```python
from build123d import *

# Parameters (mm, degrees)
F0_W     = 20.32
F0_H     = 10.16
F1_DEPTH = 5.08
F2_W     = 10.5029
F2_H     = 10.16
F3_DEPTH = 2.54
F5_D     = 1.27
F7_R     = 2.75
F7_R_2   = 0.635
F8_DEPTH = 1.524


with BuildPart() as f1:
    # F0 (on Top) → F1 (new body)
    with BuildSketch(Plane.XY):
        Rectangle(F0_W, F0_H)
    extrude(amount=F1_DEPTH)

    # F2 (on face) → F3 (cut)
    with BuildSketch(Plane.XY.offset(5.08)):
        with Locations((-2.36855, 0)):
            Rectangle(F2_W, F2_H)
    extrude(amount=-F3_DEPTH, mode=Mode.SUBTRACT)

    # F5 (through all)
    with Locations(Plane.XY.offset(5.08)):
        with Locations((6.35, 1.27), (6.35, -1.27)):
            Hole(F5_D / 2)

    # F7 (on face) → F8 (cut)
    with BuildSketch(Plane(origin=(0, 0, 0), x_dir=(1, 0, 0), z_dir=(0, 0, -1))):
        with Locations((6.35, 0)):
            Circle(F7_R)
        with Locations((6.35, -1.27)):
            Circle(F7_R_2, mode=Mode.SUBTRACT)
        with Locations((6.35, 1.27)):
            Circle(F7_R_2, mode=Mode.SUBTRACT)
    extrude(amount=-F8_DEPTH, mode=Mode.SUBTRACT)


solid = f1.part
```
CAD build for the part. Positions are in the model's coordinates, mm. A direction names the side the tool comes from. Give positions to 0.01 mm unless a question says otherwise; leave off trailing zeros. Write each loop counter-clockwise with the first axis right and the second up, starting at its lowest first coordinate (ties: lowest second). Pieces come first, ordered by that corner, then holes. Notation, with made-up numbers: M 28.25,24.25 L 61.25,24.25 A22 cw 61.25,62.25 Z; hole C 53.5,-23.5 d9. An arc over 180 degrees is marked long. Return JSON: item names as keys, results as strings. Group by question number.
(1) 3-axis set-ups, long thin cutter, end or side, ignore diameter. For faces 5 (the face through (-10.16, 0, 3)), 6 (the face through (-2, 0, 2.54)), 7 (the face through (3.6, -0.1, 0.8)): which of +Z, -Z, +X, -X, +Y, -Y reach the whole face in a straight line?
(2) Band-saw the part on A-A (z = 3). Give the cut face in (x, y) (3 decimals).
(3) Flat gauge pins, fed straight in: pin 1 Ø4.5 at (x, y) = (6, 0) entering from -Z; pin 2 Ø5 at (x, y) = (-2.5, 0) entering from +Z; pin 3 Ø1.1 at (x, y) = (6.35, 1.27) entering from -Z. Where does each tip first touch, or does it go through?
(4) Mould opens along X. For faces 1 (the face through (6, 0, 5.08)), 2 (the face through (6.984, -1.242, 3.277)), 3 (the face through (2.883, 0, 4)), 4 (the face through (10.16, 0, 3)) say: pulls with the +X half, pulls with the -X half, needs draft (parallel to the pull), parting line crosses it, or undercut.
(5) Band-saw the part on C-C (y = 4.5). Give the cut face in (x, z).
(6) Band-saw the part on D-D (y = -1.5). Give the cut face in (x, z).
(7) Band-saw the part on B-B (x = 6.35). Give the cut face in (y, z) (3 decimals).
(8) Drill centre lines: L1, parallel to X at y = 1.25, z = 4.65; L2, parallel to Y at x = 6.35, z = 2.85 (3 decimals); L3, parallel to X at y = 0, z = 0.6. Where is each one in solid material? Low to high. Write a range as [from, to].
Entries:
{
 "1": {"face 5": "+Z, -Z, -X, +Y, -Y", "face 6": "+Z, +Y, -Y", "face 7": "-Z"},
 "2": {"outline": "M -10.16,-5.08 L -7.62,-5.08 L -7.62,5.08 L -10.16,5.08 Z; M 2.883,-5.08 L 10.16,-5.08 L 10.16,5.08 L 2.883,5.08 Z; hole C 6.35,-1.27 d1.27; hole C 6.35,1.27 d1.27"},
 "3": {"pin 1": "stops at z = 1.52", "pin 2": "stops at z = 2.54", "pin 3": "passes through"},
 "4": {"face 1": "needs draft", "face 2": "undercut", "face 3": "undercut", "face 4": "pulls with the +X half"},
 "5": {"outline": "M -10.16,0 L 10.16,0 L 10.16,5.08 L 2.88,5.08 L 2.88,2.54 L -7.62,2.54 L -7.62,5.08 L -10.16,5.08 Z"},
 "6": {"outline": "M -10.16,0 L 4.05,0 L 4.05,1.52 L 5.76,1.52 L 5.76,5.08 L 2.88,5.08 L 2.88,2.54 L -7.62,2.54 L -7.62,5.08 L -10.16,5.08 Z; M 6.94,1.52 L 8.65,1.52 L 8.65,0 L 10.16,0 L 10.16,5.08 L 6.94,5.08 Z"},
 "7": {"outline": "M -5.08,0 L -2.75,0 L -2.75,1.524 L -1.905,1.524 L -1.905,5.08 L -5.08,5.08 Z; M -0.635,1.524 L 0.635,1.524 L 0.635,5.08 L -0.635,5.08 Z; M 1.905,1.524 L 2.75,1.524 L 2.75,0 L 5.08,0 L 5.08,5.08 L 1.905,5.08 Z"},
 "8": {"L1": "x = [-10.16, -7.62], [2.88, 5.72], [6.98, 10.16]", "L2": "y = [-5.08, -1.905], [-0.635, 0.635], [1.905, 5.08]", "L3": "x = [-10.16, 3.6], [9.1, 10.16]"}
}
